CAD build for the part. Positions are in the model's coordinates, mm. Face numbers are marked on the shaded views. A direction names the side the tool comes from. Give positions to 0.01 mm unless a question says otherwise; leave off trailing zeros. Loops run counter-clockwise (first coordinate to the right, second up) from the corner with the lowest first, then second, coordinate; pieces in that order, holes last. Notation, with made-up numbers: M 84.25,83 L 109.25,83 A24 cw 109.25,111 Z; hole C -28.75,-25.75 d1. An arc over 180 degrees is marked long. Answer as CSV lines item,"result".
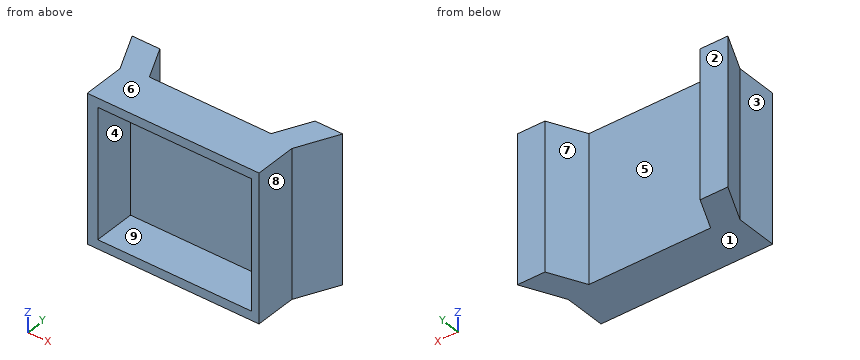
```python
from build123d import *

# Parameters (mm, degrees)
F1_DEPTH = 53.007968
F2_W     = 62
F2_H     = 53.007968
F2_W_2   = 55.406839
F2_H_2   = 46.501182
F3_DEPTH = 15


with BuildPart() as f1:
    # F0 (on Top) → F1 (new body)
    with BuildSketch(Plane.XY):
        Polygon((-1.481589, 0), (0, 0), (60.518411, 0), (67.518411, 14.453191), (57.518411, 14.453191), (51.487055, 2), (7.549767, 2), (1.518411, 14.453191), (-8.481589, 14.453191), align=None)
    extrude(amount=F1_DEPTH)

    # F2 (on face) → F3 (join)
    with BuildSketch(Plane.XZ):
        with Locations((29.518411, 26.503984)):
            Rectangle(F2_W, F2_H)
        with Locations((30.017025, 26.519272)):
            Rectangle(F2_W_2, F2_H_2, mode=Mode.SUBTRACT)
    extrude(amount=F3_DEPTH)


solid = f1.part
```
Q1. Cut at B-B (z = 19). Write the cut outline in (x, y), and give its area (3 significant figures).
Solution:
outline,"M -8.48,14.45 L -1.48,0 L -1.48,-15 L 2.31,-15 L 2.31,0 L 57.72,0 L 57.72,-15 L 60.52,-15 L 60.52,0 L 67.52,14.45 L 57.52,14.45 L 51.49,2 L 7.55,2 L 1.52,14.45 Z"
area,"474 mm²"
Q2. Cut at C-C (x = 50). Write the cut outline in (y, z), and give its area (3 significant figures).
Solution:
outline,"M -15,0 L 2,0 L 2,53.01 L -15,53.01 L -15,49.77 L 0,49.77 L 0,3.27 L -15,3.27 Z"
area,"204 mm²"
Q3. Wall check: line 1 (X direction, y = -7.25, z = 29); line 2 (Z direction, x = 16.5, y = -5); line 3 (X direction, y = 3.5, z = 47). Give the ranges that are in metal, low to high. Write a range as [from, to].
Solution:
line 1,"x = [-1.48, 2.31], [57.72, 60.52]"
line 2,"z = [0, 3.27], [49.77, 53.01]"
line 3,"x = [-3.18, 6.82], [52.21, 62.21]"
Q4. Mould opens along X. For the marked faces 6, 7, 8 and 9 say: released by +X, released by -X, zero draft, split by the parting line, or undercut.
Solution:
face 6,"zero draft"
face 7,"undercut"
face 8,"released by +X"
face 9,"undercut"
Q5. Which spindle directions (+Z, -Z, +X, -X, +Y, -Y) get a long thin tool onto all of the face, cutting with end or side? Do the marked faces 1, 2, 3, 4 and 5. Say none if no direction does.
Solution:
face 1,"-Z, +X, -X, +Y, -Y"
face 2,"+Z, -Z, +X, -X, +Y"
face 3,"+Z, -Z, -X, -Y"
face 4,"-Y"
face 5,"+Z, -Z, +Y"
Q6. Cut at A-A (y = -5.25). Write the cut outline in (x, z).
Solution:
outline,"M -1.48,0 L 60.52,0 L 60.52,53.01 L -1.48,53.01 Z; hole M 2.31,3.27 L 57.72,3.27 L 57.72,49.77 L 2.31,49.77 Z"
Q7. Cut at D-D (y = 9.25). Write the cut outline in (x, z).
Solution:
outline,"M -5.96,0 L 4.04,0 L 4.04,53.01 L -5.96,53.01 Z; M 55,0 L 65,0 L 65,53.01 L 55,53.01 Z"
Q8. Pin check, flat tips, straight feed: P1, Ø7.5, axis at x = 20, y = -10, coming from the -Z side; P2, Ø4, axis at y = 2, z = 40, coming from the -X side; P3, Ø12, axis at y = -4.5, z = 31, coming from the +X side; P4, Ø4, axis at x = 48.5, z = 33.5, coming from the +Y side. Stop position of each tip, or through.
Solution:
P1,"stops at z = 0"
P2,"stops at x = -3.42"
P3,"stops at x = 61.24"
P4,"stops at y = 2"
